Design review of the part shown in the three views and the two pictorial views. Dimensions are in mm from the part's minimum x, y and z. A direction names the side the tool comes from. Round coordinates to 2 decimals unless told otherwise and drop trailing zeros. Write each loop counter-clockwise with the first axis right and the second up, starting at its lowest first coordinate (ties: lowest second). Pieces come first, ordered by that corner, then holes. Notation, with made-up numbers: (46.25, 18) -> (94.25, 18) arc R30 cw to (94.25, 43) -> close; hole circle Ø1 at (44.25, -12). An arc over 180 degrees is marked (long way). One line per question, with ' | ' between items. Start each with the question number.
1) Consider section A-A (x = 8). Give the boundary of the cut face in (y, z).
2) Consider section C-C (x = 11.5). Give the boundary of the cut face in (y, z), then the cut area to 3 significant figures.
3) Consider section D-D (y = 5.5). Give the boundary of the cut face in (x, z).
4) Consider section B-B (z = 8). Give the boundary of the cut face in (x, y).
5) Insertion check: pin 1 Ø1 at (x, y) = (5, 4) entering from +Z; pin 2 Ø1 at (y, z) = (6, 2) entering from -X. Each pin has a flat end and moves straight along its axis. Give the tip position at first contact, or say it passes through.
6) For the marked faces 4 and 5, list the 3-axis set-ups (+Z, -Z, +X, -X, +Y, -Y) from which the entire face can be reached by the end or side of a thin tool; tool diameter is ignored.
7) For probe 1 along Y at (x, z) = (5.75, 1.75); probe 2 along X at (y, z) = (3, 8); probe 3 along Z at (x, y) = (10.25, 5.5), list the stretches that pass through material, from the lowest coordinate up.
8) Mouldability with a two-part tool opening along X and no side actions: class the marked faces 1, 2 and 3 as +X half, -X half, draft (parallel to the pull), parting line (faces both ways), or undercut.
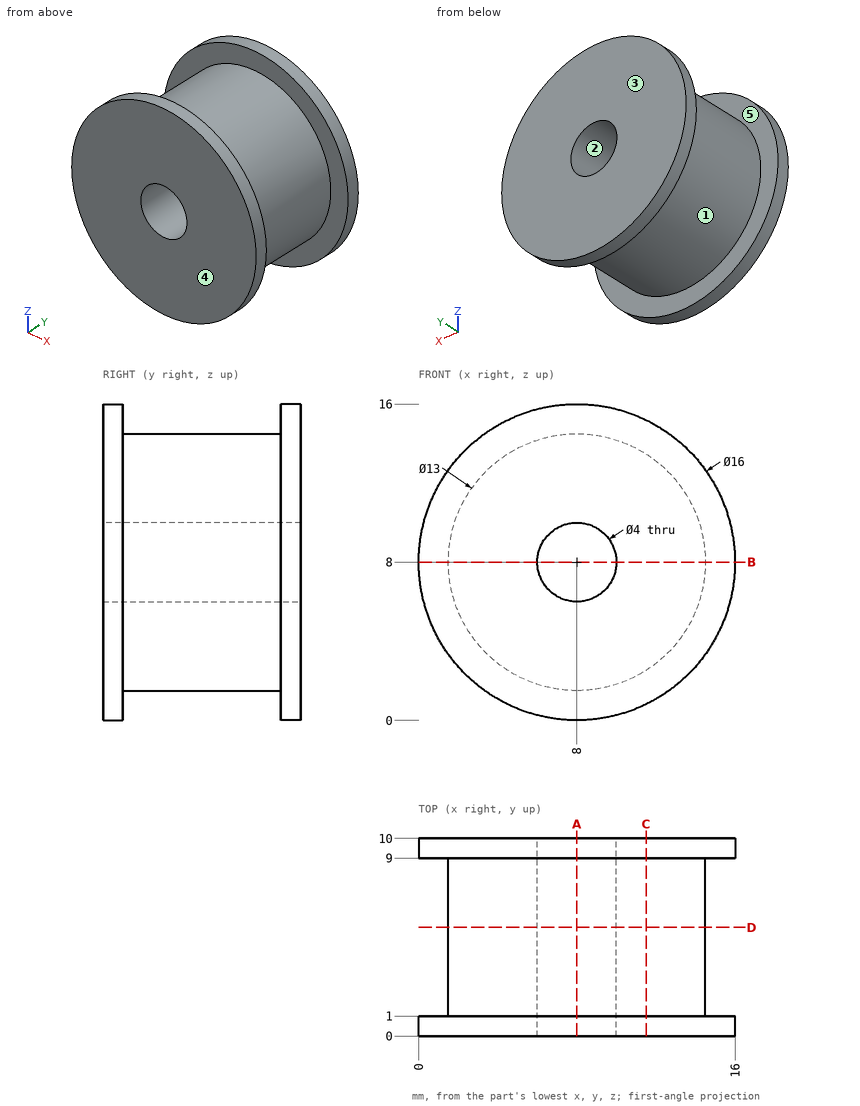
From the geometry:
1) outline: (0, 0) -> (1, 0) -> (1, 1.5) -> (9, 1.5) -> (9, 0) -> (10, 0) -> (10, 6) -> (0, 6) -> close; (0, 10) -> (10, 10) -> (10, 16) -> (9, 16) -> (9, 14.5) -> (1, 14.5) -> (1, 16) -> (0, 16) -> close
2) outline: (0, 0.81) -> (1, 0.81) -> (1, 2.52) -> (9, 2.52) -> (9, 0.81) -> (10, 0.81) -> (10, 15.19) -> (9, 15.19) -> (9, 13.48) -> (1, 13.48) -> (1, 15.19) -> (0, 15.19) -> close | area: 116 mm2
3) outline: circle Ø13 at (8, 8); hole circle Ø4 at (8, 8)
4) outline: (0, 0) -> (6, 0) -> (6, 10) -> (0, 10) -> (0, 9) -> (1.5, 9) -> (1.5, 1) -> (0, 1) -> close; (10, 0) -> (16, 0) -> (16, 1) -> (14.5, 1) -> (14.5, 9) -> (16, 9) -> (16, 10) -> (10, 10) -> close
5) pin 1: stops at z = 14 | pin 2: stops at x = 4.54
6) face 4: +Z, -Z, +X, -X, -Y | face 5: none
7) probe 1: y = 0 to 1, 9 to 10 | probe 2: x = 1.5 to 6, 10 to 14.5 | probe 3: z = 1.9 to 14.1
8) face 1: parting line | face 2: undercut | face 3: draft
